Can you work these out from the model? Positions are in its coordinate system, mm. Round coordinates to 2 decimals unless told otherwise and drop trailing zeros. Order: outer loops, then holes, each group sorted by start corner. A loop starts at its lowest first (then second) coordinate and runs counter-clockwise, first axis right, second up.
Q1. If we section it at C-C (y = 10.5): Please give me the cut outline in (x, z), plus the area to 3 significant figures.
Q2. If I drill on line 1 (X direction, y = 12.25, z = 0); line 2 (Y direction, x = -4, z = -1.75); line 3 (X direction, y = 1.5, z = 4), over which ranges is the centre line in solid material (lowest first)?
Q3. If we section it at B-B (x = 0): Please give me the cut outline in (y, z), plus the area to 3 significant figures.
Q4. If we section it at A-A (z = 0): Please give me the cut outline in (x, y), plus the area to 3 significant figures.
Q5. Will these pins go through, and if not, where does the flat tip stop? P1, Ø1, axis at x = -2, y = 3, coming from the -Z side; P2, Ø4, axis at x = -5, y = 9.5, coming from the +Z side; P3, Ø7.5, axis at x = 0, z = 0, coming from the +Y side; P4, Ø1.5, axis at x = -4, y = 7.5, coming from the -Z side.
Q6. We'd pull the mould along Z, two halves only. Please class faces 1 (the face through (-3.71, 1.48, 4.84)), 2 (the face through (-3.01, 15, 3.01)), 3 (the face through (-6.834, 7.395, -1.517)): pulls with the +Z half, pulls with the -Z half, needs draft (parallel to the pull), parting line crosses it, or undercut.
Q7. If we section it at D-D (x = 5): Please give me the cut outline in (y, z), plus the area to 3 significant figures.
from build123d import *

# Parameters (mm, degrees)
SKETCH1_R           = 7
BOSS_EXTRUDE3_DEPTH = 15
SKETCH4_R           = 4.1
CUT_EXTRUDE1_DEPTH  = 16
SKETCH5_R           = 6.1
CUT_EXTRUDE2_DEPTH  = 3


with BuildPart() as part:
    # Sketch1 → Boss-Extrude3 (new body)
    with BuildSketch(Plane(origin=(0, 0, 0), x_dir=(1, 0, 0), z_dir=(0, 1, 0))):
        with Locations(Location((0, 0, 0), (0, 0, 270))):  # turned: the seam where the file's is
            Circle(SKETCH1_R)
    extrude(amount=BOSS_EXTRUDE3_DEPTH)

    # Sketch4 → Cut-Extrude1 (cut, through all)
    with BuildSketch(Plane(origin=(0, 15, 0), x_dir=(1, 0, 0), z_dir=(0, 1, 0))):
        with Locations(Location((0, 0, 0), (0, 0, 270))):  # turned: the seam where the file's is
            Circle(SKETCH4_R)
    extrude(amount=-CUT_EXTRUDE1_DEPTH, mode=Mode.SUBTRACT)

    # Sketch5 → Cut-Extrude2 (cut)
    with BuildSketch(Plane.XZ):
        with Locations(Location((0, 0, 0), (0, 0, 270))):  # turned: the seam where the file's is
            Circle(SKETCH5_R)
    extrude(amount=-CUT_EXTRUDE2_DEPTH, mode=Mode.SUBTRACT)


solid = part.part
Solution:
1. outline: circle Ø14 at (0, 0); hole circle Ø8.2 at (0, 0)
1. area: 101 mm2
2. line 1: x = -7 to -4.1, 4.1 to 7
2. line 2: y = 3 to 15
2. line 3: x = -5.74 to -4.61, 4.61 to 5.74
3. outline: (0, -7) - (15, -7) - (15, -4.1) - (3, -4.1) - (3, -6.1) - (0, -6.1) - close; (0, 6.1) - (3, 6.1) - (3, 4.1) - (15, 4.1) - (15, 7) - (0, 7) - close
3. area: 75.0 mm2
4. outline: (-7, 0) - (-6.1, 0) - (-6.1, 3) - (-4.1, 3) - (-4.1, 15) - (-7, 15) - close; (4.1, 3) - (6.1, 3) - (6.1, 0) - (7, 0) - (7, 15) - (4.1, 15) - close
4. area: 75.0 mm2
5. P1: stops at z = -6.84
5. P2: stops at z = 6.32
5. P3: passes through
5. P4: stops at z = -6.2
6. face 1: undercut
6. face 2: needs draft
6. face 3: parting line crosses it
7. outline: (0, -4.9) - (15, -4.9) - (15, 4.9) - (0, 4.9) - (0, 3.49) - (3, 3.49) - (3, -3.49) - (0, -3.49) - close
7. area: 126 mm2
